Build history of the part. All positions in model axes, mm. Give positions to 0.01 mm unless a question says otherwise; leave off trailing zeros. Order: outer loops, then holes, each group sorted by start corner. A loop starts at its lowest first (then second) coordinate and runs counter-clockwise, first axis right, second up. Notation, with made-up numbers: (17.5, 71) -> (59.5, 71) arc R22 ccw to (59.5, 79) -> close; hole circle Ø3 at (57, 48.25). An arc over 180 degrees is marked (long way). Use a Markdown table: item, result. Add a question column.
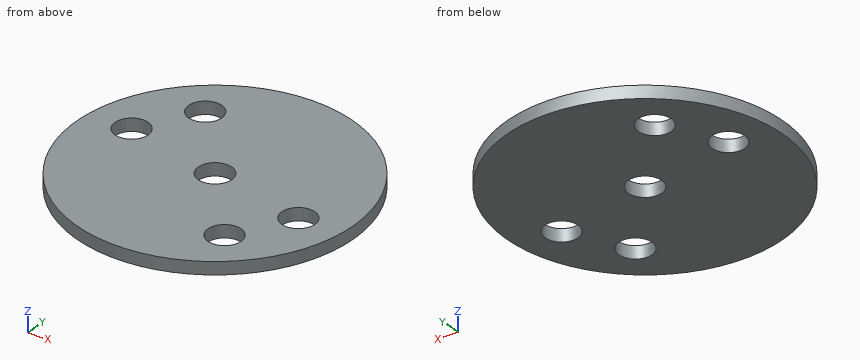
Autodesk Inventor part; units mm, degrees
ref_plane "YZ Plane" through (0, 0, 0) normal (1, 0, 0) x (0, 1, 0)
ref_plane "XZ Plane" through (0, 0, 0) normal (0, 1, 0) x (-1, 0, 0)
ref_plane "XY Plane" through (0, 0, 0) normal (0, 0, 1) x (1, 0, 0)
sketch "main" plane through (0, 0, 0) normal (0, 0, 1) x (1, 0, 0)
  circle A0 centre (-3.5355, 3.6269) radius 17.4625
  arc A1 (-12.4711, 11.0953) -> (-10.1649, 11.3129) centre (-11.4711, 12.8274) ccw
  circle A2 centre (4.4001, -5.7121) radius 2.0955
  circle A3 centre (8.5065, 1.4036) radius 2.0955
  circle A4 centre (-11.482, 12.9439) radius 2.0955
  circle A5 centre (-15.5775, 5.8503) radius 2.0955
  circle A6 centre (-3.5355, 3.6269) radius 2.1209
  point P0 (-4.7735, 4.9064)
  point P1 (3.0939, -4.059)
  point P2 (5.4001, -3.8415)
  dimension "d0" = 4.191
  dimension "d1" = 34.925
  dimension "d2" = 4.191
  dimension "d3" = 4.191
  dimension "d4" = 4.191
  dimension "d5" = 4.2418
sketch "Sketch1" plane through (0, 0, 0) normal (0, 0, 1) x (1, 0, 0)
  circle A0 centre (0, 0) radius 17.4625
  arc A1 (-8.9356, 7.4684) -> (-6.6294, 7.686) centre (-7.9356, 9.2004) ccw
  circle A2 centre (7.9356, -9.3391) radius 2.0955
  circle A3 centre (12.042, -2.2234) radius 2.0955
  circle A4 centre (-7.9465, 9.317) radius 2.0955
  circle A5 centre (-12.042, 2.2234) radius 2.0955
  circle A6 centre (0, 0) radius 2.1209
extrude "Extrusion1" add sketch "Sketch1" along normal blind 1.5875 contours A0 | A4 A1
properties part number "2in_flex_wheel_hub" material "Acetal Resin, White"
(1) Band-saw the part on D-D on x = -11.5. Give the cut face in (y, z), plus the area to 3 significant figures.
(2) Band-saw the part on C-C on z = 0.6. Give the cut face in (x, y) (1 decimal), plus the area to 3 significant figures.
(3) Pin check, flat tips, straight feed: pin 1 Ø5 at (x, y) = (-12.04, 2.22) entering from +Z; pin 2 Ø4 at (x, y) = (0, 0) entering from +Z. Stop position of each tip, or through.
(4) Band-saw the part on A-A on x = 0. Give the cut face in (y, z).
(5) Wall check: probe 1 along Y at (x, z) = (0, 0.3); probe 2 along X at (y, z) = (-0.5, 0.95); probe 3 along X at (y, z) = (8, 0.85). Give the ranges that are in metal, low to high.
(6) Band-saw the part on B-B on y = -1.5. Give the cut face in (x, z).
Response:
| question | item | result |
|---|---|---|
| 1 | outline | (-13.14, 0) -> (0.2, 0) -> (0.2, 1.59) -> (-13.14, 1.59) -> close; (4.25, 0) -> (13.14, 0) -> (13.14, 1.59) -> (4.25, 1.59) -> close |
| 1 | area | 35.3 mm² |
| 2 | outline | circle Ø34.9 at (0, 0); hole circle Ø4.2 at (-12, 2.2); hole circle Ø4.2 at (-7.9, 9.3); hole circle Ø4.2 at (0, 0); hole circle Ø4.2 at (7.9, -9.3); hole circle Ø4.2 at (12, -2.2) |
| 2 | area | 889 mm² |
| 3 | pin 1 | stops at z = 1.59 |
| 3 | pin 2 | passes through |
| 4 | outline | (-17.46, 0) -> (-2.12, 0) -> (-2.12, 1.59) -> (-17.46, 1.59) -> close; (2.12, 0) -> (17.46, 0) -> (17.46, 1.59) -> (2.12, 1.59) -> close |
| 5 | probe 1 | y = -17.46 to -2.12, 2.12 to 17.46 |
| 5 | probe 2 | x = -17.46 to -2.06, 2.06 to 10.85, 13.23 to 17.46 |
| 5 | probe 3 | x = -15.52 to -9.58, -6.32 to 15.52 |
| 6 | outline | (-17.4, 0) -> (-1.5, 0) -> (-1.5, 1.59) -> (-17.4, 1.59) -> close; (1.5, 0) -> (10.08, 0) -> (10.08, 1.59) -> (1.5, 1.59) -> close; (14.01, 0) -> (17.4, 0) -> (17.4, 1.59) -> (14.01, 1.59) -> close |
